```python
from build123d import *

# Parameters (mm, degrees)
SKETCH1_R          = 0.5
EXTRUDE1_DEPTH     = 0.508
EXTRUDE1_2_DEPTH   = 0.508
SKETCH2_W          = 2
SKETCH2_H          = 29.1
EXTRUDE2_DEPTH     = 1.5
SKETCH3_W          = 28.1
SKETCH3_H          = 29.1
EXTRUDE3_DEPTH     = 2.9
SKETCH4_W          = 27.082087072
SKETCH4_H          = 2.272405007
CUT_EXTRUDE1_DEPTH = 26.3
SKETCH5_W          = 26.233061925
SKETCH5_H          = 1.7432148
EXTRUDE4_DEPTH     = 32.5


with BuildPart() as part:
    # Sketch1 → Extrude1 (new body)
    with BuildSketch(Plane.XY):
        Circle(SKETCH1_R)
    extrude(amount=-EXTRUDE1_DEPTH)



with BuildPart() as body_2:
    # Sketch1 → Extrude1 2 (new body)
    with BuildSketch(Plane.XY):
        with Locations((26, 0)):
            Circle(SKETCH1_R)
    extrude(amount=-EXTRUDE1_2_DEPTH)


with BuildPart() as part_1:
    add(part.part)

    add(body_2.part)  # Extrude2 merges body 2
    # Sketch2 → Extrude2 (add)
    with BuildSketch(Plane.XY):
        with Locations((0, -11.75)):
            Rectangle(SKETCH2_W, SKETCH2_H)
        with Locations((26, -11.75)):
            Rectangle(SKETCH2_W, SKETCH2_H)
    extrude(amount=EXTRUDE2_DEPTH)

    # Sketch3 → Extrude3 (add)
    with BuildSketch(Plane.XY.offset(1.5)):
        with Locations((13.05, -11.75)):
            Rectangle(SKETCH3_W, SKETCH3_H)
    extrude(amount=EXTRUDE3_DEPTH)

    # Sketch4 → Cut-Extrude1 (cut)
    with BuildSketch(Plane.XZ.offset(26.3)):
        with Locations((13.034435582, 2.89542949)):
            Rectangle(SKETCH4_W, SKETCH4_H)
    extrude(amount=-CUT_EXTRUDE1_DEPTH, mode=Mode.SUBTRACT)

    # Sketch5 → Extrude4 (add)
    with BuildSketch(Plane.XZ):
        with Locations((13.116530963, 2.879865071)):
            Rectangle(SKETCH5_W, SKETCH5_H)
    extrude(amount=EXTRUDE4_DEPTH)


solid = part_1.part
```
The model under review builds one solid part; all positions refer to its coordinate system, in mm. A direction names the side the tool comes from. Round coordinates to 2 decimals unless told otherwise and drop trailing zeros. Order: outer loops, then holes, each group sorted by start corner. A loop starts at its lowest first (then second) coordinate and runs counter-clockwise, first axis right, second up.
Item 1: For pin 1 (1.2 mm diameter, centred on y = -6, z = 0.5, fed in from +X); pin 2 (13 mm diameter, centred on x = 11, y = -11.5, fed in from -Z); pin 3 (0.6 mm diameter, centred on x = 0.5, y = -17.5, fed in from -Z), all flat-tipped, find the tip position at first contact; note any pin that passes through.
Working result:
pin 1: stops at x = 27
pin 2: stops at z = 1.5
pin 3: stops at z = 0
Item 2: To check wall thickness, follow probe 1 along X at (y, z) = (-11, 3); probe 2 along Z at (x, y) = (4, -14.5); probe 3 along Z at (x, y) = (0.5, -13). State the ranges of each line that lie inside material, in increasing order.
Working result:
probe 1: x = -1 to -0.51, 0 to 26.23, 26.58 to 27.1
probe 2: z = 1.5 to 1.76, 2.01 to 3.75, 4.03 to 4.4
probe 3: z = 0 to 1.76, 2.01 to 3.75, 4.03 to 4.4
Item 3: Draft analysis for pull direction Z (two halves, no side actions). For faces 4 (the flat face through (0, 0, -0.508)), 5 (the flat face through (26.575, -13, 3)), 6 (the cylindrical face through (-0.108, -0.488, -0.25)), state which applies: released by +Z, released by -Z, zero draft, split by the parting line, or undercut.
Working result:
face 4: released by -Z
face 5: undercut
face 6: zero draft
Item 4: Add section B-B, the plane z = 3.1. State the section outline as (x, y) points.
Working result:
outline: (-1, -26.3) - (-0.51, -26.3) - (-0.51, 0) - (0, 0) - (0, -32.5) - (26.23, -32.5) - (26.23, 0) - (26.58, 0) - (26.58, -26.3) - (27.1, -26.3) - (27.1, 2.8) - (-1, 2.8) - close
Item 5: Add section A-A, the plane y = -11.5. State the section outline as (x, z) points, and give its area (3 significant figures).
Working result:
outline: (-1, 0) - (1, 0) - (1, 1.5) - (25, 1.5) - (25, 0) - (27, 0) - (27, 1.5) - (27.1, 1.5) - (27.1, 4.4) - (-1, 4.4) - close; (0, 2.01) - (26.23, 2.01) - (26.23, 3.75) - (0, 3.75) - close; hole (-0.51, 1.76) - (26.58, 1.76) - (26.58, 4.03) - (-0.51, 4.03) - close
area: 71.7 mm2
Item 6: Add section D-D, the plane y = -27. State the section outline as (x, z) points.
Working result:
outline: (0, 2.01) - (26.23, 2.01) - (26.23, 3.75) - (0, 3.75) - close
Item 7: Machinability: for faces 1 (the flat face through (13, -12, 1.5)), 2 (the cylindrical face through (26.477, 0.15, -0.25)), 3 (the flat face through (27, -12, 1)), which of the approach directions +Z, -Z, +X, -X, +Y, -Y give a long, thin tool a straight path to every point of the face, cutting with its end or side? Answer none if there is none.
Working result:
face 1: -Z, +Y, -Y
face 2: -Z
face 3: -Z, +X, +Y, -Y
Item 8: Add section C-C, the plane x = 9.75. State the section outline as (y, z) points.
Working result:
outline: (-32.5, 2.01) - (0, 2.01) - (0, 1.76) - (-26.3, 1.76) - (-26.3, 1.5) - (2.8, 1.5) - (2.8, 4.4) - (-26.3, 4.4) - (-26.3, 4.03) - (0, 4.03) - (0, 3.75) - (-32.5, 3.75) - close
